Geometry check sheet. Reference: the model listing, model coordinates, mm. Face numbers are marked on the shaded views. Give positions to 0.01 mm unless a question says otherwise; leave off trailing zeros. Write each loop counter-clockwise with the first axis right and the second up, starting at its lowest first coordinate (ties: lowest second). Pieces come first, ordered by that corner, then holes. Notation, with made-up numbers: (51, 23.5) - (62, 23.5) arc R17 cw to (62, 49.5) - close; hole circle Ø11 at (27, 79.25). An arc over 180 degrees is marked (long way). Use a Markdown table: item, result.
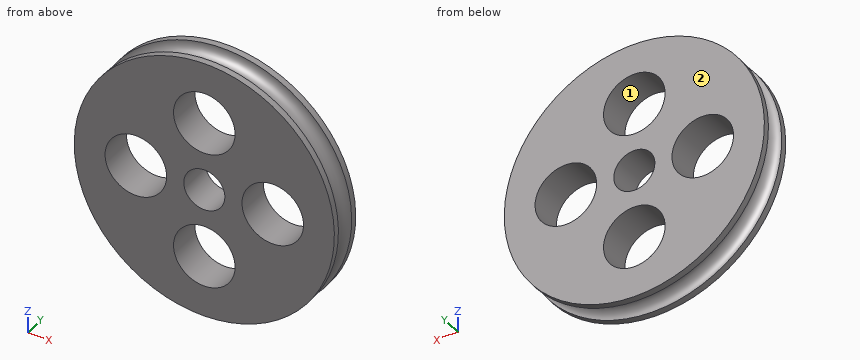
```python
from build123d import *

# Parameters (mm, degrees)
ESQUISSE2_R             = 4.5
ENL_V_MAT_EXTRU_1_DEPTH = 28.331300737


with BuildPart() as part:
    # Esquisse1 → Révolution1 (revolve)
    with BuildSketch(Plane.XY, mode=Mode.PRIVATE) as r_volution1_sk:
        with BuildLine():
            Line((-19, 0), (-3, 0))
            Line((-3, 0), (-3, 5))
            Line((-3, 5), (-19, 5))
            Line((-19, 5), (-19, 4.05))
            ThreePointArc((-19, 4.05), (-17.45, 2.5), (-19, 0.95))
            Line((-19, 0.95), (-19, 0))
        make_face()
    revolve(r_volution1_sk.sketch.rotate(Axis((0, 0, 0), (0, 1, 0)), 270), axis=Axis((0, 0, 0), (0, 1, 0)))

    # Esquisse2 → Enlèv. mat.-Extru.1 (cut, through all)
    with BuildSketch(Plane(origin=(0, 0, 0), x_dir=(-1, 0, 0), z_dir=(0, -1, 0))):
        with Locations(Location((0, -10, 0), (0, 0, 90))):
            Circle(ESQUISSE2_R)
        with Locations(Location((-10, 0, 0), (0, 0, 90))):
            Circle(ESQUISSE2_R)
        with Locations(Location((0, 10, 0), (0, 0, 90))):
            Circle(ESQUISSE2_R)
        with Locations(Location((10, 0, 0), (0, 0, 90))):
            Circle(ESQUISSE2_R)
    extrude(amount=-ENL_V_MAT_EXTRU_1_DEPTH, mode=Mode.SUBTRACT)


solid = part.part
```
1) Material ranges on L1, parallel to X at y = 0.6, z = 1; L2, parallel to X at y = 2.7, z = 0; L3, parallel to Z at x = 8.5, y = 3.7, recorded low to high. Write a range as from..to.
Working result:
| item | result |
|---|---|
| L1 | x = -18.97..-14.39, -5.61..-2.83, 2.83..5.61, 14.39..18.97 |
| L2 | x = -17.46..-14.5, -5.5..-3, 3..5.5, 14.5..17.46 |
| L3 | z = -15.89..-4.24, 4.24..15.89 |
2) Section check C-C on y = 0.5. Record the boundary of the cut face in (x, z).
Working result:
| item | result |
|---|---|
| outline | circle Ø38 at (0, 0); hole circle Ø9 at (-10, 0); hole circle Ø9 at (0, -10); hole circle Ø9 at (0, 10); hole circle Ø6 at (0, 0); hole circle Ø9 at (10, 0) |
3) Section check A-A on x = 0. Record the boundary of the cut face in (y, z).
Working result:
| item | result |
|---|---|
| outline | (0, -19) - (0.95, -19) arc R1.55 cw to (4.05, -19) - (5, -19) - (5, -14.5) - (0, -14.5) - close; (0, -5.5) - (5, -5.5) - (5, -3) - (0, -3) - close; (0, 3) - (5, 3) - (5, 5.5) - (0, 5.5) - close; (0, 14.5) - (5, 14.5) - (5, 19) - (4.05, 19) arc R1.55 cw to (0.95, 19) - (0, 19) - close |
4) Mould release check, pull along X, two halves, no side actions. Record for the marked faces 1 and 2: pulls with the +X half, pulls with the -X half, needs draft (parallel to the pull), parting line crosses it, or undercut.
Working result:
| item | result |
|---|---|
| face 1 | undercut |
| face 2 | needs draft |
5) Section check D-D on z = 4. Count the separate pieces of the cut face and the enclosed holes in it, then the cut area to 3 significant figures.
Working result:
| item | result |
|---|---|
| separate pieces | 3 |
| enclosed holes | 0 |
| area | 137 mm² |
6) Section check B-B on z = 0. Record the boundary of the cut face in (x, y).
Working result:
| item | result |
|---|---|
| outline | (-19, 0) - (-14.5, 0) - (-14.5, 5) - (-19, 5) - (-19, 4.05) arc R1.55 cw to (-19, 0.95) - close; (-5.5, 0) - (-3, 0) - (-3, 5) - (-5.5, 5) - close; (3, 0) - (5.5, 0) - (5.5, 5) - (3, 5) - close; (14.5, 0) - (19, 0) - (19, 0.95) arc R1.55 cw to (19, 4.05) - (19, 5) - (14.5, 5) - close |
